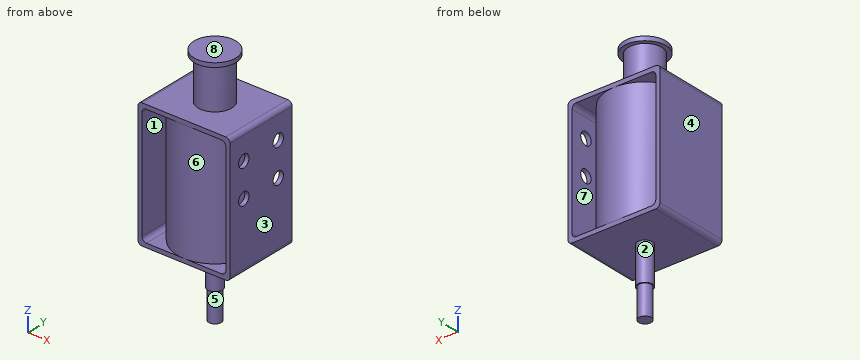
Autodesk Inventor part; units mm, degrees
ref_plane "YZ Plane" through (0, 0, 0) normal (1, 0, 0) x (0, 1, 0)
ref_plane "XZ Plane" through (0, 0, 0) normal (0, 1, 0) x (-1, 0, 0)
ref_plane "XY Plane" through (0, 0, 0) normal (0, 0, 1) x (1, 0, 0)
sketch "Sketch1" plane through (0, 0, 0) normal (0, 1, 0) x (-1, 0, 0)
  line L0 (-11, 14.2) -> (-11, -14.2)
  line L1 (-10, -15.2) -> (10, -15.2)
  line L2 (11, -14.2) -> (11, 14.2)
  line L3 (10, 15.2) -> (-10, 15.2)
  line L4 (-11, 15.2) -> (11, -15.2) construction
  line L5 (-11, -15.2) -> (11, 15.2) construction
  line L6 (-10, 13.2) -> (-10, -13.2)
  line L7 (-9, -14.2) -> (9, -14.2)
  line L8 (10, -13.2) -> (10, 13.2)
  line L9 (9, 14.2) -> (-9, 14.2)
  line L10 (-10, 14.2) -> (10, -14.2) construction
  line L11 (-10, -14.2) -> (10, 14.2) construction
  arc A0 (11, 14.2) -> (10, 15.2) centre (10, 14.2) ccw
  arc A1 (10, 13.2) -> (9, 14.2) centre (9, 13.2) ccw
  arc A2 (9, -14.2) -> (10, -13.2) centre (9, -13.2) ccw
  arc A3 (10, -15.2) -> (11, -14.2) centre (10, -14.2) ccw
  arc A4 (-10, -13.2) -> (-9, -14.2) centre (-9, -13.2) ccw
  arc A5 (-11, -14.2) -> (-10, -15.2) centre (-10, -14.2) ccw
  arc A6 (-10, 15.2) -> (-11, 14.2) centre (-10, 14.2) ccw
  arc A7 (-9, 14.2) -> (-10, 13.2) centre (-9, 13.2) ccw
  point P0 (0, 0)
  dimension "d0" = 30.4
  dimension "d1" = 22
  dimension "d2" = 28.4
  dimension "d3" = 20
  dimension "d4" = 1
  dimension "d5" = 1
extrude "Extrusion1" add sketch "Sketch1" along normal blind 18
sketch "Sketch3" plane through (-9, 0, -14.2) normal (0, 0, 1) x (1, 0, 0)
  line L0 (9, 0) -> (9, 9)
  circle A0 centre (9, 9) radius 9
  dimension "d12" = 9
  dimension "d13" = 18
extrude "Extrusion3" add sketch "Sketch3" along normal up to surface (28.4 mm away)
sketch "Sketch4" plane through (-10, 0, 15.2) normal (0, 0, 1) x (1, 0, 0)
  circle A0 centre (10, 9) radius 4
  point P0 (10, 0)
  dimension "d16" = 8
extrude "Extrusion4" add sketch "Sketch4" along normal blind 10
sketch "Sketch5" plane through (0, 9, 25.2) normal (0, 0, 1) x (1, 0, 0)
  circle A0 centre (0, 0) radius 5
  point P0 (0, -9)
  dimension "d19" = 10
extrude "Extrusion5" add sketch "Sketch5" along normal blind 1
sketch "Sketch7" plane through (10, 0, -15.2) normal (0, 0, -1) x (-1, 0, 0)
  line L0 (10, 9) -> (10, 0)
  circle A0 centre (10, 9) radius 1.75
  dimension "d22" = 3.5
extrude "Extrusion6" add sketch "Sketch7" along normal blind 9
sketch "Sketch8" plane through (11, 0, 14.2) normal (1, 0, 0) x (0, 0, -1)
  line L0 (-1, 0) -> (-1, 18)
  line L1 (-1, 9) -> (5.5, 9)
  line L2 (5.5, 9) -> (5.5, 14)
  line L3 (5.5, 14) -> (5.5, 4)
  line L4 (5.5, 4) -> (13.5, 4)
  line L5 (13.5, 4) -> (13.5, 14)
  circle A0 centre (5.5, 14) radius 1.5
  circle A1 centre (13.5, 14) radius 1.5
  circle A2 centre (13.5, 4) radius 1.5
  circle A3 centre (5.5, 4) radius 1.5
  point P0 (14.2, 0)
  dimension "d25" = 6.5
  dimension "d26" = 5
  dimension "d27" = 10
  dimension "d28" = 8
  dimension "d29" = 3
  dimension "d30" = 3
  dimension "d31" = 3
  dimension "d32" = 3
extrude "Extrusion7" cut sketch "Sketch8" against normal blind 2
sketch "Sketch9" plane through (0, 9, -24.2) normal (0, 0, -1) x (-1, 0, 0)
  circle A0 centre (0, 0) radius 1.5
  point P0 (0, -9)
  dimension "d35" = 3
extrude "Extrusion8" add sketch "Sketch9" along normal blind 7
thread "Thread1"
properties part number "Solenoid"
Check sheet for the modelled part. Datum: model origin and axes. Units: mm. Face numbers are marked on the shaded views. A direction names the side the tool comes from. Round coordinates to 2 decimals unless told otherwise and drop trailing zeros. Order: outer loops, then holes, each group sorted by start corner. A loop starts at its lowest first (then second) coordinate and runs counter-clockwise, first axis right, second up. Notation, with made-up numbers: (27.5, 71) -> (51.5, 71) arc R23 cw to (51.5, 86) -> close; hole circle Ø5 at (-37, -25.75). An arc over 180 degrees is marked (long way). One line per item, written item: value. Start each with the question number.
Q1. Gauge pin test, flat ends, axial feed: pin 1 Ø2.5 at (x, y) = (-4.5, 14) entering from -Z; pin 2 Ø2 at (x, z) = (6.5, 3.5) entering from +Y; pin 3 Ø2.5 at (x, y) = (6, 6.5) entering from +Z. Record the tip position at first contact, or that the pin passes through.
Q2. Thickness scan on line 1 (Y direction, x = 10.6, z = 0.7); line 2 (Z direction, x = -4, y = 11.5); line 3 (Z direction, x = 10.65, y = 4). Record the ranges inside material, lowest first.
Q3. Set-up check for the marked faces 4, 5, 6, 7 and 8: record each of +Z, -Z, +X, -X, +Y, -Y from which the full face is reachable in a straight line by a thin tool's end or side.
Q4. Mould release check, pull along X, two halves, no side actions. Record for the marked faces 1, 2 and 3: pulls with the +X half, pulls with the -X half, needs draft (parallel to the pull), parting line crosses it, or undercut.
Q5. Cross-section at D-D (z = -18.5). Record the boundary of the cut face in (x, y).
Q6. Cross-section at A-A (z = -6). Record the boundary of the cut face in (x, y).
Q7. Cross-section at C-C (x = -6.5). Record the boundary of the cut face in (y, z), and give its area (3 significant figures).
Q8. Cross-section at B-B (z = 8.7). Record the boundary of the cut face in (x, y), and give its area (3 significant figures).
Completed:
1. pin 1: stops at z = -15.2
1. pin 2: stops at y = 16.12
1. pin 3: stops at z = 15.2
2. line 1: y = 0 to 2.5, 5.5 to 12.5, 15.5 to 18
2. line 2: z = -15.2 to 15.2, 25.2 to 26.2
2. line 3: z = -14.96 to -0.8, 2.2 to 7.2, 10.2 to 14.96
3. face 4: +Z, -Z, -X, +Y, -Y
3. face 5: -Z
3. face 6: none
3. face 7: +Y, -Y
3. face 8: +Z, +X, -X, +Y, -Y
4. face 1: undercut
4. face 2: parting line crosses it
4. face 3: pulls with the +X half
5. outline: circle Ø3.5 at (0, 9)
6. outline: (-11, 0) -> (-10, 0) -> (-10, 18) -> (-11, 18) -> close; circle Ø18 at (0, 9); (10, 0) -> (11, 0) -> (11, 18) -> (10, 18) -> close
7. outline: (0, -15.2) -> (18, -15.2) -> (18, -14.2) -> (15.22, -14.2) -> (15.22, 14.2) -> (18, 14.2) -> (18, 15.2) -> (0, 15.2) -> (0, 14.2) -> (2.78, 14.2) -> (2.78, -14.2) -> (0, -14.2) -> close
7. area: 390 mm²
8. outline: (-11, 0) -> (-10, 0) -> (-10, 18) -> (-11, 18) -> close; circle Ø18 at (0, 9); (10, 0) -> (11, 0) -> (11, 2.5) -> (10, 2.5) -> close; (10, 5.5) -> (11, 5.5) -> (11, 12.5) -> (10, 12.5) -> close; (10, 15.5) -> (11, 15.5) -> (11, 18) -> (10, 18) -> close
8. area: 284 mm²
